```python
from build123d import *

# Parameters (mm, degrees)
SKETCH_1_W          = 38
SKETCH_1_H          = 3.6
EXTRUDE_1_DEPTH     = 157
SKETCH_2_R          = 1.6
EXTRUDE_2_DEPTH     = 3
CUT_EXTRUDE_1_DEPTH = 172.997042126


with BuildPart() as part:
    # 草图1 → 凸台-拉伸1 (new body)
    with BuildSketch(Plane(origin=(0, 0, 0), x_dir=(0, 0, -1), z_dir=(1, 0, 0))):
        Rectangle(SKETCH_1_W, SKETCH_1_H)
    extrude(amount=EXTRUDE_1_DEPTH)

    # 草图2 → 凸台-拉伸2 (add)
    # profile 1 of 2: a face of its own
    with BuildSketch(Plane(origin=(0, 1.8, 0), x_dir=(1, 0, 0), z_dir=(0, 1, 0))):
        with BuildLine():
            Line((36.3, -19), (10, -19))
            Line((10, -19), (0, -19))
            Line((0, -19), (0, -70.15))
            Line((0, -70.15), (10, -70.15))
            Line((10, -70.15), (10, -49))
            Line((10, -49), (10, -44.575))
            ThreePointArc((10, -44.575), (23.15, -35.125450458), (36.3, -44.575))
            Line((36.3, -44.575), (36.3, -49))
            Line((36.3, -49), (36.3, -70.15))
            Line((36.3, -70.15), (46.3, -70.15))
            Line((46.3, -70.15), (46.3, -19))
            Line((46.3, -19), (36.3, -19))
        make_face()
        with Locations(Location((5, -66.15, 0), (0, 0, 270))):
            Circle(SKETCH_2_R, mode=Mode.SUBTRACT)
        with Locations(Location((41.3, -66.15, 0), (0, 0, 270))):
            Circle(SKETCH_2_R, mode=Mode.SUBTRACT)
    # profile 2 of 2: a face of its own
    with BuildSketch(Plane(origin=(0, 1.8, 0), x_dir=(1, 0, 0), z_dir=(0, 1, 0))):
        with BuildLine():
            Line((120.7, -49), (120.7, -44.575))
            ThreePointArc((120.7, -44.575), (133.85, -35.125450458), (147, -44.575))
            Line((147, -44.575), (147, -49))
            Line((147, -49), (147, -70.15))
            Line((147, -70.15), (157, -70.15))
            Line((157, -70.15), (157, -19))
            Line((157, -19), (147, -19))
            Line((147, -19), (120.7, -19))
            Line((120.7, -19), (110.7, -19))
            Line((110.7, -19), (110.7, -70.15))
            Line((110.7, -70.15), (120.7, -70.15))
            Line((120.7, -70.15), (120.7, -49))
        make_face()
        with Locations(Location((115.7, -66.15, 0), (0, 0, 270))):
            Circle(SKETCH_2_R, mode=Mode.SUBTRACT)
        with Locations(Location((152, -66.15, 0), (0, 0, 270))):
            Circle(SKETCH_2_R, mode=Mode.SUBTRACT)
    extrude(amount=-EXTRUDE_2_DEPTH)

    # 草图4 → 切除-拉伸1 (cut, through all)
    with BuildSketch(Plane(origin=(0, 1.8, 0), x_dir=(1, 0, 0), z_dir=(0, 1, 0))):
        Polygon((105, 19.2), (94.6, 19.2), (94.6, 11.9), (84.6, 11.9), (84.6, 4), (105, 4), align=None)
        Polygon((145, 19.2), (134.6, 19.2), (134.6, 11.9), (124.6, 11.9), (124.6, 4), (145, 4), align=None)
    extrude(amount=-CUT_EXTRUDE_1_DEPTH, mode=Mode.SUBTRACT)


solid = part.part
```
Work out the finished part from the listing and answer in its coordinate system (mm). A direction names the side the tool comes from. Coordinates: 2 decimals unless noted, no trailing zeros. Write each loop counter-clockwise with the first axis right and the second up, starting at its lowest first coordinate (ties: lowest second). Pieces come first, ordered by that corner, then holes. Notation, with made-up numbers: (-10.5, 77.25) - (48.5, 77.25) arc R29 ccw to (48.5, 114.25) - close; hole circle Ø10 at (-38.75, 73). An arc over 180 degrees is marked (long way). Answer as a JSON object with one key per item and string values.
Q1. Find section A-A (z = 53). Write down the section's boundary in (x, y).
Results list:
{"outline": "(0, -1.2) - (10, -1.2) - (10, 1.8) - (0, 1.8) - close; (36.3, -1.2) - (46.3, -1.2) - (46.3, 1.8) - (36.3, 1.8) - close; (110.7, -1.2) - (120.7, -1.2) - (120.7, 1.8) - (110.7, 1.8) - close; (147, -1.2) - (157, -1.2) - (157, 1.8) - (147, 1.8) - close"}
Q2. Find section C-C (y = 0.95). State how many separate pieces and enclosed holes the cut face has, plus the area to 3 significant figures.
Results list:
{"separate pieces": "1", "enclosed holes": "4", "area": "8,490 mm^2"}
Q3. Which of the six approach directions +Z, -Z, +X, -X, +Y, -Y give full straight-line access (tool end or side, diameter ignored) to faces 4 (the flat face through (145, 0, -11)), 5 (the flat face through (36.3, 0, 57)), 6 (the flat face through (130, 0, -11.9))?
Results list:
{"face 4": "-Z, +Y, -Y", "face 5": "+Z, +Y, -Y", "face 6": "+Y, -Y"}
Q4. Given pin 1 Ø3.5 at (x, z) = (5, 66.15) entering from -Y; pin 2 Ø1.8 at (x, y) = (97.5, 0.5) entering from -Z; pin 3 Ø1.1 at (x, y) = (91, 1) entering from +Z, each flat-ended and moving along its own axis, determine where each tip first touches the part or whether it passes through.
Results list:
{"pin 1": "stops at y = -1.2", "pin 2": "stops at z = -4", "pin 3": "stops at z = 19"}
Q5. For a pull along Z with two mould halves and no side action, classify faces 1 (the flat face through (124.6, 0, -8)), 2 (the flat face through (105, 0, -11)), 3 (the flat face through (120, 0, -19)) as pulls with the +Z half, pulls with the -Z half, needs draft (parallel to the pull), parting line crosses it, or undercut.
Results list:
{"face 1": "undercut", "face 2": "needs draft", "face 3": "pulls with the -Z half"}
Q6. Find section B-B (x = 152). Write down the section's boundary in (y, z).
Results list:
{"outline": "(-1.8, -19) - (1.8, -19) - (1.8, 64.55) - (-1.2, 64.55) - (-1.2, 19) - (-1.8, 19) - close; (-1.2, 67.75) - (1.8, 67.75) - (1.8, 70.15) - (-1.2, 70.15) - close"}
Q7. Consider L1, parallel to Z at x = 115.7, y = 0.4; L2, parallel to X at y = 1.05, z = 29; L3, parallel to Z at x = 89.5, y = 0.85. Determine where each line is inside the solid, lowest interval first. Write a range as from..to.
Results list:
{"L1": "z = -19..64.55, 67.75..70.15", "L2": "x = 0..46.3, 110.7..157", "L3": "z = -19..-11.9, -4..19"}
